```python
from build123d import *

# Parameters (mm, degrees)
F0_R     = 11.90625
F0_R_2   = 6.35
F1_DEPTH = 0.127
F3_R     = 0.9921875
F4_DEPTH = 3.81
F5_COUNT = 18


with BuildPart() as f1:
    # F0 (on Top) → F1 (new body, symmetric)
    with BuildSketch(Plane.XY):
        Circle(F0_R)
        Circle(F0_R_2, mode=Mode.SUBTRACT)
    extrude(amount=F1_DEPTH, both=True)

    # F3 (on offset) → F4 (join)
    with BuildSketch(Plane.XZ.offset(10.668)):
        with Locations((0, 0.1984869643)):
            Circle(F3_R)
    extrude(amount=-F4_DEPTH)

    # F5: F1 ×18 about axis
    f5_axis = Axis((0, 0, 0), (0, 0, -1))


with BuildPart() as f1_1:
    add(f1.part)
    for i in range(1, F5_COUNT):
        add(f1.part.rotate(f5_axis, i * 360 / F5_COUNT))


solid = f1_1.part
```
Build history of the part. All positions in model axes, mm. A direction names the side the tool comes from. Give positions to 0.01 mm unless a question says otherwise; leave off trailing zeros. Loops run counter-clockwise (first coordinate to the right, second up) from the corner with the lowest first, then second, coordinate; pieces in that order, holes last.
Item 1: Flat gauge pins, fed straight in: pin 1 (0.9 mm diameter, centred on x = 0, z = 1, fed in from -Y); pin 2 (1 mm diameter, centred on y = 2, z = 1, fed in from +X); pin 3 (0.9 mm diameter, centred on x = -0.5, z = 1, fed in from +Y). Where does each tip first touch, or does it go through?
Answers follow:
pin 1: stops at y = -10.67
pin 2: stops at x = 10.57
pin 3: stops at y = 10.67
Item 2: Drill centre lines: line 1 (Y direction, x = 0, z = 0.05); line 2 (Y direction, x = 0.75, z = -0.35); line 3 (X direction, y = -8.75, z = -0.4). Where is each one in solid material? Low to high.
Answers follow:
line 1: y = -11.91 to -6.35, 6.35 to 11.91
line 2: y = -10.67 to -6.86, 6.86 to 10.67
line 3: x = -4.03 to -2.34, -0.79 to 0.79, 2.34 to 4.03
Item 3: Which spindle directions (+Z, -Z, +X, -X, +Y, -Y) get a long thin tool onto all of the face, cutting with end or side? Do faces 1 (the face through (4.418, 5.245, -0.382)), 2 (the face through (-10.504, 1.866, 0.548)), 3 (the face through (2.33, -6.45, 0.55)), 4 (the face through (9.23, -5.35, 0.55)). Say none if no direction does.
Answers follow:
face 1: -Z
face 2: +Z, -X, +Y
face 3: +Z
face 4: +Z, +X, -Y
Item 4: Slice it at B-B, the plane z = -0.45. Give the number of separate pieces and of enclosed holes in the cut face, and give its area (3 significant figures).
Answers follow:
separate pieces: 18
enclosed holes: 0
area: 103 mm2
Item 5: Pull direction Y, two halves, no side cores. Call faces 5 (the face through (3.636, -10.029, 0.548)), 6 (the face through (-7.621, -4.38, -0.794)), 7 (the face through (0.017, 8.79, -0.794)): released by +Y, released by -Y, zero draft, split by the parting line, or undercut.
Answers follow:
face 5: released by -Y
face 6: undercut
face 7: zero draft
Item 6: Slice it at A-A, the plane x = 0. List the corners of the cut face in (y, z), and give its area (3 significant figures).
Answers follow:
outline: (-11.91, -0.13) - (-10.67, -0.13) - (-10.67, -0.79) - (-6.86, -0.79) - (-6.86, -0.13) - (-6.35, -0.13) - (-6.35, 0.13) - (-6.86, 0.13) - (-6.86, 1.19) - (-10.67, 1.19) - (-10.67, 0.13) - (-11.91, 0.13) - close; (6.35, -0.13) - (6.86, -0.13) - (6.86, -0.79) - (10.67, -0.79) - (10.67, -0.13) - (11.91, -0.13) - (11.91, 0.13) - (10.67, 0.13) - (10.67, 1.19) - (6.86, 1.19) - (6.86, 0.13) - (6.35, 0.13) - close
area: 16.0 mm2
